from build123d import *

# Parameters (mm, degrees)
SKETCH_1_R          = 2.6356377382591165
SKETCH_1_R_2        = 2.6356377382590894
SKETCH_1_R_3        = 2.6356377382590765
SKETCH_1_R_4        = 2.635637738259072
EXTRUDE_1_DEPTH     = 5
EXTRUDE_START       = -50
EXTRUDE_2_DEPTH     = 50
FILLET_1_R          = 3
EXTRUDE_START_2     = -70
EXTRUDE_3_DEPTH     = 70
FILLET_2_R          = 3
EXTRUDE_4_DEPTH     = 70
SKETCH_5_W          = 89.0633311885125
SKETCH_5_H          = 295.3242731829526
CUT_EXTRUDE_1_DEPTH = 275.0000000000001


with BuildPart() as part:
    # 스케치1 → 보스-돌출1 (new body)
    with BuildSketch(Plane.XY):
        with BuildLine():
            Line((-161.90972688439834, -132.69604313286513), (-19.251249440125157, -86.34349397662291))
            Line((-19.251249440125157, -86.34349397662291), (21.87942689934009, -86.34349397662294))
            Line((21.87942689934009, -86.34349397662294), (21.87942689934009, -48.00694505649064))
            Line((21.87942689934009, -48.00694505649064), (-33.73868544416714, -48.00694505649063))
            ThreePointArc((-33.73868544416714, -48.00694505649063), (-98.53802186230143, 23.53498808064043), (-187.05476471538051, 62.031590942583435))
            Line((-187.05476471538051, 62.031590942583435), (-187.05476471538051, 96.21524094975992))
            Line((-187.05476471538051, 96.21524094975992), (-225.3913136355128, 96.21524094975996))
            Line((-225.3913136355128, 96.21524094975996), (-225.3913136355128, 64.75798291501623))
            Line((-225.3913136355128, 64.75798291501623), (-222.25805676193863, 64.75798291501623))
            ThreePointArc((-222.25805676193863, 64.75798291501623), (-98.36294899741762, 21.51708345847385), (-18.952715979656908, -82.95199333393413))
            ThreePointArc((-18.952715979656908, -82.95199333393413), (-19.008196216614675, -84.1549577478759), (-19.915396046499477, -84.94691097033295))
            Line((-19.915396046499477, -84.94691097033295), (-162.3835926892786, -131.2376341463548))
            Line((-162.3835926892786, -131.2376341463548), (-161.90972688439834, -132.69604313286513))
        make_face()
        with Locations((-215.8071764054797, 86.63110371972729)):
            Circle(SKETCH_1_R, mode=Mode.SUBTRACT)
        with Locations((-196.63890194541358, 86.6311037197273)):
            Circle(SKETCH_1_R_2, mode=Mode.SUBTRACT)
        with Locations((12.295289669307014, -76.75935674658983)):
            Circle(SKETCH_1_R_3, mode=Mode.SUBTRACT)
        with Locations((12.295289669307014, -57.5910822865237)):
            Circle(SKETCH_1_R_4, mode=Mode.SUBTRACT)
    extrude(amount=EXTRUDE_1_DEPTH)

    # 스케치2 → 보스-돌출2 (add)
    with BuildSketch(Plane.XY.offset(5).offset(EXTRUDE_START)):
        with BuildLine():
            Line((-161.90972688439834, -132.69604313286513), (-19.25124944012515, -86.34349397662291))
            Line((-19.251249440125157, -86.34349397662291), (-17.716653821091654, -86.34349397662291))
            ThreePointArc((-17.71665382109279, -86.34349397662707), (-18.32795901714934, -84.64529234814141), (-18.952715979656915, -82.95199333393413))
            ThreePointArc((-18.95271597965692, -82.95199333393413), (-19.008196216614667, -84.1549577478759), (-19.915396046499477, -84.94691097033295))
            Line((-19.915396046499477, -84.94691097033295), (-162.3835926892786, -131.2376341463548))
            Line((-162.3835926892786, -131.2376341463548), (-161.90972688439834, -132.69604313286513))
        make_face()
        with BuildLine():
            ThreePointArc((-18.952715979656915, -82.95199333393413), (-18.32795901714934, -84.64529234814141), (-17.71665382109279, -86.34349397662707))
            Line((-17.716653821091654, -86.34349397662291), (-16.089863152321414, -86.34349397662291))
            ThreePointArc((-16.08986315232295, -86.34349397662834), (-24.029465542915716, -66.76788414274672), (-33.7386854441672, -48.006945056490636))
            ThreePointArc((-33.7386854441672, -48.006945056490636), (-98.53802186230149, 23.53498808064043), (-187.0547647153805, 62.03159094258342))
            ThreePointArc((-187.0547647153805, 62.03159094258342), (-206.13076342964123, 65.02753015483808), (-225.39131363551047, 66.40614702590713))
            Line((-225.3913136355128, 66.4061470259071), (-225.3913136355128, 64.87202248366495))
            ThreePointArc((-225.3913136355129, 64.87202248366495), (-223.82448876300626, 64.82039980470964), (-222.25805676193858, 64.75798291501621))
            ThreePointArc((-222.25805676193858, 64.75798291501621), (-98.36294899741759, 21.51708345847382), (-18.952715979656915, -82.95199333393413))
        make_face()
    extrude(amount=EXTRUDE_2_DEPTH)

    # 필렛1
    # the kernel refuses this fillet: 3 mm, written as the material it takes off along each edge
    with BuildSketch(Plane(origin=(-16.089863152324853, -86.34349397662284, -55.26319649463599), x_dir=(-0.3411564748454367, 0.9400065210789948, 0), z_dir=(0, 0, 1))) as fillet_1_piece_1:
        with BuildLine():
            CenterArc((4.078395273634998, 2.9998795453949634), FILLET_1_R, 180.53774443113053, 89.97569611298013)
            Line((1.0785274015705548, 2.971723726182023), (0, 0))
            ThreePointArc((0, 0), (2.052639298925323, -0.00919714593498524), (4.105278597850862, -9e-17))
        make_face()
    extrude(amount=55.26319649463599, mode=Mode.SUBTRACT)

    # 스케치3 → 보스-돌출3 (add)
    with BuildSketch(Plane.XY.offset(5).offset(EXTRUDE_START_2)):
        with BuildLine():
            Line((-19.25124944012515, -86.34349397662291), (-161.90972688439834, -132.69604313286513))
            Line((-161.90972688439834, -132.69604313286513), (-161.14752471177883, -135.0418602115354))
            Line((-161.14752471177883, -135.0418602115354), (-13.733764686030042, -87.14422608341849))
            ThreePointArc((-13.73376468603007, -87.1442260834185), (-13.872485363120319, -86.74373244280719), (-14.011940562426247, -86.34349397662855))
            Line((-14.011940562424655, -86.34349397662291), (-19.251249440125157, -86.34349397662291))
        make_face()
        with BuildLine():
            Line((-33.738685444167196, -48.00694505649064), (-31.477883861441427, -48.00694505649064))
            ThreePointArc((-31.477883861440404, -48.00694505648765), (-97.09546483661316, 24.91254341428484), (-187.05476471538535, 64.03086517268349))
            Line((-187.05476471538051, 64.03086517268437), (-187.05476471538051, 62.03159094258343))
            ThreePointArc((-187.0547647153805, 62.03159094258345), (-98.53802186230146, 23.53498808064043), (-33.738685444167174, -48.00694505649062))
        make_face()
        with BuildLine():
            Line((-162.3835926892786, -131.2376341463548), (-161.90972688439834, -132.69604313286513))
            Line((-161.90972688439834, -132.69604313286513), (-19.25124944012515, -86.34349397662291))
            Line((-19.251249440125157, -86.34349397662291), (-14.011940562424655, -86.34349397662291))
            ThreePointArc((-14.011940562426247, -86.34349397662855), (-21.86923355209842, -66.77626462229537), (-31.477883861440404, -48.00694505648765))
            Line((-31.477883861441427, -48.00694505649064), (-33.738685444167196, -48.00694505649064))
            ThreePointArc((-33.738685444167174, -48.00694505649062), (-98.53802186230146, 23.53498808064043), (-187.0547647153805, 62.03159094258345))
            Line((-187.05476471538051, 62.03159094258343), (-187.05476471538051, 64.03086517268437))
            ThreePointArc((-187.05476471538535, 64.03086517268349), (-206.13235139969905, 67.00089307897522), (-225.3913136355111, 68.36755070296968))
            Line((-225.3913136355128, 68.36755070296962), (-225.3913136355128, 64.75798291501623))
            Line((-225.3913136355128, 64.75798291501623), (-222.2580567619386, 64.75798291501621))
            ThreePointArc((-222.2580567619386, 64.75798291501624), (-98.36294899741762, 21.51708345847382), (-18.952715979656915, -82.95199333393413))
            ThreePointArc((-18.95271597965692, -82.95199333393413), (-19.008196216614667, -84.1549577478759), (-19.915396046499477, -84.94691097033295))
            Line((-19.915396046499477, -84.94691097033295), (-162.3835926892786, -131.2376341463548))
        make_face()
    extrude(amount=EXTRUDE_3_DEPTH)

    # 필렛2
    fillet_2_edges = [part.edges().sort_by_distance(p)[0] for p in [
        (-13.733764686030042, -87.14422608341849, -30),
    ]]
    fillet(fillet_2_edges, radius=FILLET_2_R)

    # 스케치4 → 보스-돌출4 (add)
    with BuildSketch(Plane.XY.offset(5)):
        with BuildLine():
            ThreePointArc((-16.659298654257338, -88.09478969169395), (-15.531728736228363, -87.42760572202484), (-14.796031724606808, -86.34349397662291))
            ThreePointArc((-14.796031724606877, -86.34349397662292), (-22.25453577932595, -66.79124041647023), (-31.477883861438727, -48.006945056490636))
            ThreePointArc((-31.4778838614387, -48.006945056490636), (-97.09546483660972, 24.912543414282396), (-187.05476471538054, 64.03086517268255))
            ThreePointArc((-187.0547647153805, 64.03086517268252), (-206.09486736019076, 67.8503266656956), (-225.3913136355128, 70.03228816057364))
            Line((-225.3913136355128, 70.03228816057364), (-225.3913136355128, 64.75798291501623))
            Line((-225.3913136355128, 64.75798291501623), (-222.2580567619386, 64.75798291501621))
            ThreePointArc((-222.2580567619386, 64.75798291501624), (-98.36294899741762, 21.51708345847382), (-18.952715979656915, -82.95199333393413))
            ThreePointArc((-18.95271597965692, -82.95199333393413), (-19.008196216614667, -84.1549577478759), (-19.915396046499477, -84.94691097033295))
            Line((-19.915396046499477, -84.94691097033295), (-162.3835926892786, -131.2376341463548))
            Line((-162.3835926892786, -131.2376341463548), (-161.14752471177886, -135.0418602115354))
            Line((-161.14752471177886, -135.0418602115354), (-16.659298654257327, -88.09478969169395))
        make_face()
    extrude(amount=EXTRUDE_4_DEPTH)

    # 스케치5 → 컷-돌출1 (cut)
    with BuildSketch(Plane.ZY.offset(225.3913136355128)):
        with Locations((-44.53166559425625, -79.29458588850659)):
            Rectangle(SKETCH_5_W, SKETCH_5_H)
    extrude(amount=-CUT_EXTRUDE_1_DEPTH, mode=Mode.SUBTRACT)


solid = part.part
The model under review builds one solid part; all positions refer to its coordinate system, in mm. A direction names the side the tool comes from. Round coordinates to 2 decimals unless told otherwise and drop trailing zeros. Write each loop counter-clockwise with the first axis right and the second up, starting at its lowest first coordinate (ties: lowest second). Pieces come first, ordered by that corner, then holes. Notation, with made-up numbers: M 32,78 L 75,78 A34 ccw 75,114 Z; hole C 71.25,84 d3. An arc over 180 degrees is marked long. Use a Markdown table: item, result. Add a question column.
Q1. We need section D-D, the plane x = -177.5. State the section outline as (y, z) points, plus the area to 3 significant figures.
Q2. Machinability: for faces 4 (the face through (-217.9, 85.03, 2.46)), 5 (the face through (-22.138, -67.06, 39.51)), 6 (the face through (-99.88, 22.61, 36.98)), which of the approach directions +Z, -Z, +X, -X, +Y, -Y give a long, thin tool a straight path to every point of the face, cutting with its end or side? Answer none if there is none.
Q3. We need section A-A, the plane x = -147.5. State the section outline as (y, z) points.
Q4. We need section B-B, the plane z = 24.5. State the section outline as (x, y) points, plus the area to 3 significant figures.
Q5. The part is to be moulded in two halves that separate along Y. For faces 1 (the face through (-90.152, -107.768, 36.975)), 2 (the face through (-206, 80, 5)), 3 (the face through (-205.83, 67.81, 39.51)), say which applies: pulls with the +Y half, pulls with the -Y half, needs draft (parallel to the pull), parting line crosses it, or undercut.
Q6. Insertion check: pin 1 (1.6 mm diameter, centred on x = -224, z = 41, fed in from -Y); pin 2 (5.5 mm diameter, centred on x = -4.5, z = 1.5, fed in from -Y); pin 3 (1.5 mm diameter, centred on y = -49, z = 46.5, fed in from -X). Each pin has a flat end and moves straight along its axis. Give the tip position at first contact, or say it passes through.
Q7. To check wall thickness, follow line 1 (Y direction, x = -145.5, z = 17); line 2 (Y direction, x = -82.5, z = 10); line 3 (X direction, y = -75.5, z = 51). State the ranges of each line that lie inside material, in increasing order.
Q8. We need section C-C, the plane y = -39. State the section outline as (x, z) points, plus the area to 3 significant figures.
Findings below:
| question | item | result |
|---|---|---|
| 1 | outline | M 58.32,0 L 61.92,0 L 61.92,75 L 58.32,75 Z |
| 1 | area | 270 mm² |
| 2 | face 4 | +Z, -Z |
| 2 | face 5 | +Z, +X, +Y |
| 2 | face 6 | +Z, -Z, -X |
| 3 | outline | M -130.61,0 L -126.4,0 L -126.4,75 L -130.61,75 Z; M 48.66,0 L 52.42,0 L 52.42,75 L 48.66,75 Z |
| 4 | outline | M -225.39,64.76 L -222.26,64.76 A227.53 cw -18.95,-82.95 A1.53 cw -19.92,-84.95 L -162.38,-131.24 L -161.15,-135.04 L -16.66,-88.09 A3 ccw -14.8,-86.34 A227.53 ccw -31.48,-48.01 A231.02 ccw -187.05,64.03 A227.53 ccw -225.39,70.03 Z |
| 4 | area | 1,590 mm² |
| 5 | face 1 | undercut |
| 5 | face 2 | needs draft |
| 5 | face 3 | pulls with the +Y half |
| 6 | pin 1 | stops at y = 64.76 |
| 6 | pin 2 | stops at y = -86.34 |
| 6 | pin 3 | stops at x = -35.37 |
| 7 | line 1 | y = -129.96 to -125.75, 47.85 to 51.62 |
| 7 | line 2 | y = -109.49 to -105.28, 8.87 to 13.49 |
| 7 | line 3 | x = -21.89 to -18.68 |
| 8 | outline | M -41.04,0 L -36.9,0 L -36.9,75 L -41.04,75 Z |
| 8 | area | 311 mm² |
